from build123d import *

# Parameters (mm, degrees)
SKETCH1_R           = 50.5
BOSS_EXTRUDE1_DEPTH = 5
SKETCH3_R           = 14
SKETCH3_R_2         = 1.65
BOSS_EXTRUDE2_DEPTH = 10
SKETCH6_R           = 1
CUT_EXTRUDE4_DEPTH  = 10
SKETCH5_R           = 4.835
CUT_EXTRUDE3_DEPTH  = 73.114492302
CUT_EXTRUDE10_REACH = 74.976
SKETCH12_R          = 1.7
SKETCH15_W          = 2.5
SKETCH15_H          = 10
BOSS_EXTRUDE3_DEPTH = 10
CUT_EXTRUDE11_REACH = 74.114
SKETCH13_R          = 2.2
CIRPATTERN1_COUNT   = 3


with BuildPart() as part:
    # Sketch1 → Boss-Extrude1 (new body)
    with BuildSketch(Plane(origin=(0, 0, 0), x_dir=(1, 0, 0), z_dir=(0, 1, 0))):
        with Locations(Location((0, 0, 0), (0, 0, 270))):
            Circle(SKETCH1_R)
    extrude(amount=BOSS_EXTRUDE1_DEPTH)

    # Sketch3 → Boss-Extrude2 (add)
    with BuildSketch(Plane(origin=(0, 5, 0), x_dir=(1, 0, 0), z_dir=(0, 1, 0))):
        with Locations(Location((0, 0, 0), (0, 0, 270))):
            Circle(SKETCH3_R)
        with Locations(Location((9, 0, 0), (0, 0, 270))):
            Circle(SKETCH3_R_2, mode=Mode.SUBTRACT)
        with Locations(Location((4.5, -7.794228634, 0), (0, 0, 270))):
            Circle(SKETCH3_R_2, mode=Mode.SUBTRACT)
        with Locations(Location((-4.5, -7.794228634, 0), (0, 0, 270))):
            Circle(SKETCH3_R_2, mode=Mode.SUBTRACT)
        with Locations(Location((-9, 0, 0), (0, 0, 270))):
            Circle(SKETCH3_R_2, mode=Mode.SUBTRACT)
        with Locations(Location((-4.5, 7.794228634, 0), (0, 0, 270))):
            Circle(SKETCH3_R_2, mode=Mode.SUBTRACT)
        with Locations(Location((4.5, 7.794228634, 0), (0, 0, 270))):
            Circle(SKETCH3_R_2, mode=Mode.SUBTRACT)
    extrude(amount=BOSS_EXTRUDE2_DEPTH)

    # Sketch6 → Cut-Extrude4 (cut)
    with BuildSketch(Plane(origin=(0, 5, 0), x_dir=(1, 0, 0), z_dir=(0, 1, 0))):
        with Locations(Location((18.75, 0, 0), (0, 0, 270))):
            Circle(SKETCH6_R)
        with Locations(Location((9.375, -16.237976321, 0), (0, 0, 270))):
            Circle(SKETCH6_R)
        with Locations(Location((-9.375, -16.237976321, 0), (0, 0, 270))):
            Circle(SKETCH6_R)
        with Locations(Location((-18.75, 0, 0), (0, 0, 270))):
            Circle(SKETCH6_R)
        with Locations(Location((-9.375, 16.237976321, 0), (0, 0, 270))):
            Circle(SKETCH6_R)
        with Locations(Location((9.375, 16.237976321, 0), (0, 0, 270))):
            Circle(SKETCH6_R)
    extrude(amount=-CUT_EXTRUDE4_DEPTH, mode=Mode.SUBTRACT)

    # Sketch5 → Cut-Extrude3 (cut, through all)
    with BuildSketch(Plane(origin=(0, 5, 0), x_dir=(1, 0, 0), z_dir=(0, 1, 0))):
        with Locations(Location((28, 0, 0), (0, 0, 270))):
            Circle(SKETCH5_R)
        with Locations(Location((14, -24.248711306, 0), (0, 0, 270))):
            Circle(SKETCH5_R)
        with Locations(Location((-14, -24.248711306, 0), (0, 0, 270))):
            Circle(SKETCH5_R)
        with Locations(Location((-28, 0, 0), (0, 0, 270))):
            Circle(SKETCH5_R)
        with Locations(Location((-14, 24.248711306, 0), (0, 0, 270))):
            Circle(SKETCH5_R)
        with Locations(Location((14, 24.248711306, 0), (0, 0, 270))):
            Circle(SKETCH5_R)
    extrude(amount=-CUT_EXTRUDE3_DEPTH, mode=Mode.SUBTRACT)

    # Sketch12 → Cut-Extrude10 (cut, up to next)
    with BuildSketch(Plane.XZ, mode=Mode.PRIVATE) as cut_extrude10_sk1:
        with Locations(Location((0, 42.5, 0), (0, 0, 270))):
            Circle(SKETCH12_R)
    cut_extrude10_tool1 = extrude(cut_extrude10_sk1.sketch, amount=-CUT_EXTRUDE10_REACH, mode=Mode.PRIVATE) & part.part
    cut_extrude10 = cut_extrude10_tool1.solids().sort_by_distance((0, 0, 42.5))[0]
    add(cut_extrude10, mode=Mode.SUBTRACT)

    # Sketch15 → Boss-Extrude3 (add)
    with BuildSketch(Plane.XZ.offset(-5)):
        with Locations((-4.85, 42.5)):
            Rectangle(SKETCH15_W, SKETCH15_H)
        with Locations((4.85, 42.5)):
            Rectangle(SKETCH15_W, SKETCH15_H)
    boss_extrude3 = extrude(amount=-BOSS_EXTRUDE3_DEPTH)

    # Sketch13 → Cut-Extrude11 (cut, up to next)
    with BuildSketch(Plane(origin=(0, 5, 0), x_dir=(1, 0, 0), z_dir=(0, 1, 0)), mode=Mode.PRIVATE) as cut_extrude11_sk1:
        with Locations(Location((0, 42.5, 0), (0, 0, 270))):
            Circle(SKETCH13_R)
    cut_extrude11_tool1 = extrude(cut_extrude11_sk1.sketch, amount=-CUT_EXTRUDE11_REACH, mode=Mode.PRIVATE) & part.part
    cut_extrude11 = cut_extrude11_tool1.solids().sort_by_distance((0, 5, -42.5))[0]
    add(cut_extrude11, mode=Mode.SUBTRACT)

    # CirPattern1: Cut-Extrude10, Boss-Extrude3, Cut-Extrude11 ×3 about axis
    cirpattern1_axis = Axis((0, 0, 0), (0, 1, 0))
    add([cut_extrude10.rotate(cirpattern1_axis, i * 360 / CIRPATTERN1_COUNT) for i in range(1, CIRPATTERN1_COUNT)], mode=Mode.SUBTRACT)
    add([boss_extrude3.rotate(cirpattern1_axis, i * 360 / CIRPATTERN1_COUNT) for i in range(1, CIRPATTERN1_COUNT)])
    add([cut_extrude11.rotate(cirpattern1_axis, i * 360 / CIRPATTERN1_COUNT) for i in range(1, CIRPATTERN1_COUNT)], mode=Mode.SUBTRACT)


solid = part.part
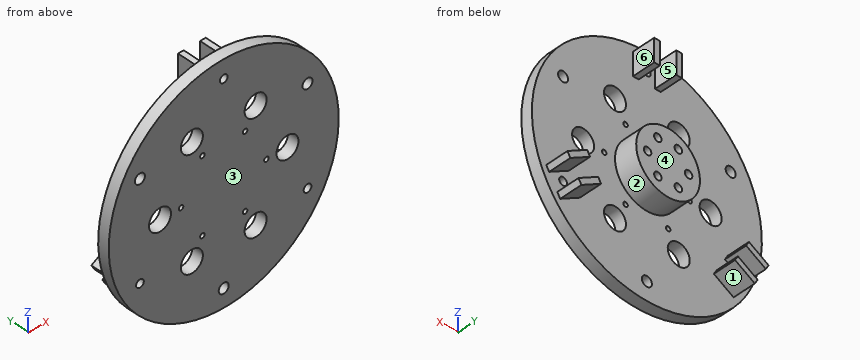
CAD build for the part. Positions are in the model's coordinates, mm. Face numbers are marked on the shaded views. A direction names the side the tool comes from. Give positions to 0.01 mm unless a question says otherwise; leave off trailing zeros. Loops run counter-clockwise (first coordinate to the right, second up) from the corner with the lowest first, then second, coordinate; pieces in that order, holes last. Notation, with made-up numbers: M -3.75,6.5 L 11.25,6.5 A25 ccw 11.25,21.5 Z; hole C -31.5,-37 d4. An arc over 180 degrees is marked long. Write each question's results on one line, items separated by ' | '.
Q1. Band-saw the part on D-D on x = 40.5. Write the cut outline in (y, z), and give its area (3 significant figures).
Geometry check:
outline: M 0,-30.17 L 5,-30.17 L 5,-19.23 L 15,-19.23 L 15,-16.34 L 5,-16.34 L 5,30.17 L 0,30.17 Z | area: 331 mm²
Q2. Which spindle directions (+Z, -Z, +X, -X, +Y, -Y) get a long thin tool onto all of the face, cutting with end or side? Do the marked faces 1, 2 and 3. Say none if no direction does.
Geometry check:
face 1: -Z, +Y | face 2: +Y | face 3: +Z, -Z, +X, -X, -Y
Q3. Mould opens along X. For the marked faces 4, 5 and 6 say: pulls with the +X half, pulls with the -X half, needs draft (parallel to the pull), parting line crosses it, or undercut.
Geometry check:
face 4: needs draft | face 5: undercut | face 6: pulls with the +X half
Q4. Probe probe 1 along X at (y, z) = (3.6, 0) (3 decimals); probe 2 along X at (y, z) = (11.5, 46.5); probe 3 along X at (y, z) = (4.5, -16.5). List the from-to ranges inside material, lowest first.
Geometry check:
probe 1: x = -50.5 to -32.835, -23.165 to -19.75, -17.75 to 17.75, 19.75 to 23.165, 32.835 to 50.5 | probe 2: x = -6.1 to -3.6, 3.6 to 6.1 | probe 3: x = -47.73 to -10.34, -8.41 to 8.41, 10.34 to 47.73
Q5. Flat gauge pins, fed straight in: P1, Ø3, axis at x = -9, z = 0, coming from the +Y side; P2, Ø8, axis at y = 7.5, z = 43.5, coming from the +X side; P3, Ø3, axis at y = 8, z = 43, coming from the -X side; P4, Ø1.6, axis at x = 18.75, z = 0, coming from the +Y side. Where does each tip first touch, or does it go through?
Geometry check:
P1: stops at y = 5 | P2: stops at x = 30.33 | P3: stops at x = -6.1 | P4: passes through
Q6. Band-saw the part on B-B on z = -42.5. Write the cut outline in (x, y), and give its area (3 significant figures).
Geometry check:
outline: M -27.28,0 L -2.2,0 L -2.2,5 L -27.28,5 Z; M 2.2,0 L 27.28,0 L 27.28,5 L 2.2,5 Z | area: 251 mm²
Q7. Band-saw the part on A-A on y = 10.25. Give the number of separate pieces and of enclosed holes in the cut face, and give its area (3 significant figures).
Geometry check:
separate pieces: 7 | enclosed holes: 6 | area: 714 mm²
